Input: part model. Units: mm. Frame: model coordinates. A direction names the side the tool comes from. Round coordinates to 2 decimals unless told otherwise and drop trailing zeros. Loops run counter-clockwise (first coordinate to the right, second up) from the corner with the lowest first, then second, coordinate; pieces in that order, holes last. Notation, with made-up numbers: (51.25, -31) -> (69.25, -31) arc R7 cw to (69.25, -23) -> close; hole circle Ø6 at (-33, 54.25). An arc over 180 degrees is marked (long way). One line per question, with ' | ' between items. Start each with the question number.
Q1. Contact query for flat-ended pins moving along their axis: P1, Ø1.4, axis at y = 0.5, z = -2.5, coming from the +X side; P2, Ø3.5, axis at x = 0, y = -8, coming from the +Z side; P3, Ø5, axis at x = -2, y = 5.5, coming from the -Z side; P4, Ø14.5, axis at x = -7, y = 5, coming from the -Z side. Output: stop coordinate, or through.
Q2. Material intervals for L1, parallel to Y at x = 0, z = 28.75; L2, parallel to X at y = 8, z = 31.5; L3, parallel to Z at x = -1.5, y = 3.5, sorted ascending.
Q3. Cut plane C-C on z = 34. Return loops of the section in (x, y), and give its area (3 significant figures).
Q4. Cut plane B-B on x = 0. Return loops of the section in (y, z) (3 decimals), and give its area (3 significant figures).
Q5. Mould query, pull axis X, two halves, no side actions, for faces 1 (the face through (-0.28, 6.73, 30.4)), 2 (the face through (0, 0, 54.2)), 3 (the face through (4.793, -1.509, 39.082)), 4 (the face through (8.4, 0, -3)). Classes: pulls with the +X half, pulls with the -X half, needs draft (parallel to the pull), parting line crosses it, or undercut.
Q6. Cut plane D-D on z = 46.5. Return loops of the section in (x, y), and give its area (3 significant figures).
Q7. Access query for faces 5 (the face through (13.926, -4.385, 18.635)), 6 (the face through (-8.4, 0, -3)), 7 (the face through (4.793, 1.509, -1.282)), 8 (the face through (8, 0, -3)), 9 (the face through (-0.91, 0.7, 47.2)). Directions: +Z, -Z, +X, -X, +Y, -Y. A direction counts if a zero-diameter tool reaches every point of the face in a straight line with its end or side. Return the directions, or none.
Q8. Cut plane A-A on y = 0. Return loops of the section in (x, z) (3 decimals), and give its area (3 significant figures).
Autodesk Inventor part; units mm, degrees
ref_plane "YZ Plane" through (0, 0, 0) normal (1, 0, 0) x (0, 1, 0)
ref_plane "XZ Plane" through (0, 0, 0) normal (0, 1, 0) x (-1, 0, 0)
ref_plane "XY Plane" through (0, 0, 0) normal (0, 0, 1) x (1, 0, 0)
sketch "スケッチ1" plane through (0, 0, 0) normal (0, 0, 1) x (1, 0, 0)
  circle A0 centre (0, 0) radius 14.6
  circle A1 centre (0, 0) radius 5.025
  line L0 (0, 0) -> (8, 0)
  line L1 (0, 0) -> (-8, 0)
  circle A2 centre (0, 0) radius 1.15
  line L2 (-8, 0) -> (-8, -1.4)
  line L3 (-8, -1.4) -> (-8, 1.4)
  line L4 (8, 0) -> (8, -1.4)
  line L5 (8, -1.4) -> (8, 1.4)
  line L6 (8.4, -1.4) -> (8.4, 1.4)
  line L7 (-8.4, 1.4) -> (-8.4, -1.4)
  line L8 (-8.4, -1.4) -> (-8, -1.4)
  line L9 (-8.4, 1.4) -> (-8, 1.4)
  line L10 (8, -1.4) -> (8.4, -1.4)
  line L11 (8, 1.4) -> (8.4, 1.4)
  dimension "d0" = 29.2
  dimension "d1" = 10.05
  dimension "d2" = 8
  dimension "d3" = 8
  dimension "d6" = 2.3
  dimension "d21" = 1.4
  dimension "d22" = 2.8
  dimension "d23" = 1.4
  dimension "d24" = 2.8
  dimension "d25" = 0.4
  dimension "d26" = 0.4
extrude "押し出し1" add sketch "スケッチ1" along normal blind 37.8 contours A0 | L0 A2 L1 A1 | L2 L8 L7 L9 L3 | A1 L1 A2 L0 | L5 L11 L6 L10 L4 | A2 L1 L0 | L0 L1 A2
extrude "押し出し2" add sketch "スケッチ1" against normal blind 2.6 contours L0 A2 L1 A1 | A1 L1 A2 L0 | A2 L1 L0 | L0 L1 A2
extrude "押し出し3" add sketch "スケッチ1" along normal blind 40.4 contours L0 A2 L1 A1 | A1 L1 A2 L0 | A2 L1 L0 | L0 L1 A2
extrude "押し出し4" add sketch "スケッチ1" along normal blind 54.2 contours A2 L1 L0 | L0 L1 A2
sketch "スケッチ2" plane through (0, 0, 37.8) normal (0, 0, 1) x (1, 0, 0)
  line L0 (0, 0) -> (0, 8)
  line L1 (0, 0) -> (0, -8)
  circle A0 centre (0, -8) radius 1.3
  circle A1 centre (0, 8) radius 1.3
  dimension "d15" = 8
  dimension "d16" = 8
  dimension "d17" = 2.6
  dimension "d18" = 2.6
extrude "押し出し5" cut sketch "スケッチ2" against normal blind 15
extrude "押し出し6" add sketch "スケッチ1" against normal blind 7 contours L2 L8 L7 L9 L3 | L5 L11 L6 L10 L4
properties part number "モーター(形だけ)"
Results:
1) P1: x = 8.4 | P2: z = 37.8 | P3: z = -2.6 | P4: z = -7
2) L1: -14.6 to -9.3, -6.7 to 6.7, 9.3 to 14.6 | L2: -12.21 to -1.3, 1.3 to 12.21 | L3: -2.6 to 40.4
3) outline: circle Ø29.2 at (0, 0); hole circle Ø2.6 at (0, -8); hole circle Ø2.6 at (0, 8) | area: 659 mm^2
4) outline: (-14.6, 0) -> (-5.025, 0) -> (-5.025, -2.6) -> (5.025, -2.6) -> (5.025, 0) -> (14.6, 0) -> (14.6, 37.8) -> (9.3, 37.8) -> (9.3, 22.8) -> (6.7, 22.8) -> (6.7, 37.8) -> (5.025, 37.8) -> (5.025, 40.4) -> (1.15, 40.4) -> (1.15, 54.2) -> (-1.15, 54.2) -> (-1.15, 40.4) -> (-5.025, 40.4) -> (-5.025, 37.8) -> (-6.7, 37.8) -> (-6.7, 22.8) -> (-9.3, 22.8) -> (-9.3, 37.8) -> (-14.6, 37.8) -> close | area: 1,110 mm^2
5) face 1: undercut | face 2: needs draft | face 3: parting line crosses it | face 4: pulls with the +X half
6) outline: circle Ø2.3 at (0, 0) | area: 4.15 mm^2
7) face 5: +Z, -Z | face 6: -Z, -X, +Y, -Y | face 7: -Z | face 8: -Z, +Y, -Y | face 9: +Z
8) outline: (-14.6, 0) -> (-8.4, 0) -> (-8.4, -7) -> (-8, -7) -> (-8, 0) -> (-5.025, 0) -> (-5.025, -2.6) -> (5.025, -2.6) -> (5.025, 0) -> (8, 0) -> (8, -7) -> (8.4, -7) -> (8.4, 0) -> (14.6, 0) -> (14.6, 37.8) -> (5.025, 37.8) -> (5.025, 40.4) -> (1.15, 40.4) -> (1.15, 54.2) -> (-1.15, 54.2) -> (-1.15, 40.4) -> (-5.025, 40.4) -> (-5.025, 37.8) -> (-14.6, 37.8) -> close | area: 1,190 mm^2
